```python
from build123d import *

# Parameters (mm, degrees)
SKETCH034_R     = 2.15
PAD006_DEPTH    = 14.6
SKETCH035_R     = 1.3
HOLE_DEPTH      = 8.7
HOLE_TIPS_R     = 1.3
SKETCH036_R     = 1.3
HOLE001_DEPTH   = 8.7
HOLE001_TIPS_R  = 1.3
SKETCH037_R     = 1.3
HOLE002_DEPTH   = 9.218881
HOLE002_TIPS_R  = 1.3
CHAMFER_SIZE    = 0.99
CHAMFER011_SIZE = 0.3


with BuildPart() as part:
    # Sketch034 → Pad006 (new body, symmetric)
    with BuildSketch(Plane.XZ):
        with BuildLine():
            Line((-9.454213, -1.414214), (-8.5, -2.368427))
            Line((-8.5, -2.368427), (-8.5, -5.5))
            Line((-8.5, -5.5), (-19, -5.5))
            Line((-19, -5.5), (-20, -4.5))
            Line((-20, -4.5), (-20, 11))
            Line((-20, 11), (-19, 12))
            Line((-19, 12), (-10, 12))
            Line((-10, 12), (-9, 11))
            Line((-9, 11), (9, 11))
            Line((9, 11), (10, 12))
            Line((10, 12), (19, 12))
            Line((19, 12), (20, 11))
            Line((20, 11), (20, -4.5))
            Line((20, -4.5), (19, -5.5))
            Line((19, -5.5), (8.5, -5.5))
            Line((8.5, -5.5), (8.5, -2.368427))
            Line((8.5, -2.368427), (9.454214, -1.414214))
            ThreePointArc((9.454214, -1.414214), (9.963946, 0.546289), (8.5, 1.946381))
            Line((8.5, 1.946381), (8.5, 4))
            ThreePointArc((8.5, 4), (8.207107, 4.707107), (7.5, 5))
            Line((7.5, 5), (-7.5, 5))
            ThreePointArc((-7.5, 5), (-8.207107, 4.707107), (-8.5, 4))
            Line((-8.5, 4), (-8.5, 1.946381))
            ThreePointArc((-8.5, 1.946381), (-9.963946, 0.546289), (-9.454213, -1.414214))
        make_face()
        with Locations((-16.700254, 5)):
            Circle(SKETCH034_R, mode=Mode.SUBTRACT)
        with Locations((16.700254, 5)):
            Circle(SKETCH034_R, mode=Mode.SUBTRACT)
    extrude(amount=PAD006_DEPTH, both=True)

    # Sketch035 → Hole (cut)
    with BuildSketch(Plane.XZ.offset(14.6)):
        with Locations((-14.679528, -1.5)):
            Circle(SKETCH035_R)
        with Locations((14.679528, -1.5)):
            Circle(SKETCH035_R)
        with Locations((0, 8)):
            Circle(SKETCH035_R)
    extrude(amount=-HOLE_DEPTH, mode=Mode.SUBTRACT)

    # Hole tips → Hole tip 1 section 0
    with BuildSketch(Plane.XZ.offset(5.9), mode=Mode.PRIVATE) as hole_tip_1_s0:
        with Locations((-14.679528, -1.5)):
            Circle(HOLE_TIPS_R)
    loft([hole_tip_1_s0.sketch, Vertex(-14.679528, -4.6, -1.5)], mode=Mode.SUBTRACT)

    # Hole tips → Hole tip 2 section 0
    with BuildSketch(Plane.XZ.offset(5.9), mode=Mode.PRIVATE) as hole_tip_2_s0:
        with Locations((14.679528, -1.5)):
            Circle(HOLE_TIPS_R)
    loft([hole_tip_2_s0.sketch, Vertex(14.679528, -4.6, -1.5)], mode=Mode.SUBTRACT)

    # Hole tips → Hole tip 3 section 0
    with BuildSketch(Plane.XZ.offset(5.9), mode=Mode.PRIVATE) as hole_tip_3_s0:
        with Locations((0, 8)):
            Circle(HOLE_TIPS_R)
    loft([hole_tip_3_s0.sketch, Vertex(0, -4.6, 8)], mode=Mode.SUBTRACT)

    # Sketch036 → Hole001 (cut)
    with BuildSketch(Plane(origin=(0, 14.6, 0), x_dir=(-1, 0, 0), z_dir=(0, 1, 0))):
        with Locations((14.679528, -1.5)):
            Circle(SKETCH036_R)
        with Locations((-14.679528, -1.5)):
            Circle(SKETCH036_R)
        with Locations((0, 8)):
            Circle(SKETCH036_R)
    extrude(amount=-HOLE001_DEPTH, mode=Mode.SUBTRACT)

    # Hole001 tips → Hole001 tip 1 section 0
    with BuildSketch(Plane(origin=(0, 5.9, 0), x_dir=(-1, 0, 0), z_dir=(0, 1, 0)), mode=Mode.PRIVATE) as hole001_tip_1_s0:
        with Locations((14.679528, -1.5)):
            Circle(HOLE001_TIPS_R)
    loft([hole001_tip_1_s0.sketch, Vertex(-14.679528, 4.6, -1.5)], mode=Mode.SUBTRACT)

    # Hole001 tips → Hole001 tip 2 section 0
    with BuildSketch(Plane(origin=(0, 5.9, 0), x_dir=(-1, 0, 0), z_dir=(0, 1, 0)), mode=Mode.PRIVATE) as hole001_tip_2_s0:
        with Locations((-14.679528, -1.5)):
            Circle(HOLE001_TIPS_R)
    loft([hole001_tip_2_s0.sketch, Vertex(14.679528, 4.6, -1.5)], mode=Mode.SUBTRACT)

    # Hole001 tips → Hole001 tip 3 section 0
    with BuildSketch(Plane(origin=(0, 5.9, 0), x_dir=(-1, 0, 0), z_dir=(0, 1, 0)), mode=Mode.PRIVATE) as hole001_tip_3_s0:
        with Locations((0, 8)):
            Circle(HOLE001_TIPS_R)
    loft([hole001_tip_3_s0.sketch, Vertex(0, 4.6, 8)], mode=Mode.SUBTRACT)

    # Sketch037 → Hole002 (cut)
    with BuildSketch(Plane.XY.offset(12)):
        with Locations((-12.5, 10)):
            Circle(SKETCH037_R)
        with Locations((12.5, 10)):
            Circle(SKETCH037_R)
        with Locations((12.5, -10)):
            Circle(SKETCH037_R)
        with Locations((-12.5, -10)):
            Circle(SKETCH037_R)
    extrude(amount=-HOLE002_DEPTH, mode=Mode.SUBTRACT)

    # Hole002 tips → Hole002 tip 1 section 0
    with BuildSketch(Plane.XY.offset(2.781119), mode=Mode.PRIVATE) as hole002_tip_1_s0:
        with Locations((-12.5, 10)):
            Circle(HOLE002_TIPS_R)
    loft([hole002_tip_1_s0.sketch, Vertex(-12.5, 10, 2)], mode=Mode.SUBTRACT)

    # Hole002 tips → Hole002 tip 2 section 0
    with BuildSketch(Plane.XY.offset(2.781119), mode=Mode.PRIVATE) as hole002_tip_2_s0:
        with Locations((12.5, 10)):
            Circle(HOLE002_TIPS_R)
    loft([hole002_tip_2_s0.sketch, Vertex(12.5, 10, 2)], mode=Mode.SUBTRACT)

    # Hole002 tips → Hole002 tip 3 section 0
    with BuildSketch(Plane.XY.offset(2.781119), mode=Mode.PRIVATE) as hole002_tip_3_s0:
        with Locations((12.5, -10)):
            Circle(HOLE002_TIPS_R)
    loft([hole002_tip_3_s0.sketch, Vertex(12.5, -10, 2)], mode=Mode.SUBTRACT)

    # Hole002 tips → Hole002 tip 4 section 0
    with BuildSketch(Plane.XY.offset(2.781119), mode=Mode.PRIVATE) as hole002_tip_4_s0:
        with Locations((-12.5, -10)):
            Circle(HOLE002_TIPS_R)
    loft([hole002_tip_4_s0.sketch, Vertex(-12.5, -10, 2)], mode=Mode.SUBTRACT)

    # Chamfer
    chamfer_edges = [part.edges().sort_by_distance(p)[0] for p in [
        (14.5, 14.6, 12),
        (-14.5, 14.6, 12),
        (-14.5, -14.6, 12),
        (14.5, -14.6, 12),
    ]]
    chamfer(chamfer_edges, length=CHAMFER_SIZE)

    # Chamfer011
    chamfer011_edges = [part.edges().sort_by_distance(p)[0] for p in [
        (-13.8, -10, 12),
        (-13.8, 10, 12),
        (11.2, 10, 12),
        (11.2, -10, 12),
        (13.379528, -14.6, -1.5),
        (-15.979528, -14.6, -1.5),
        (-1.3, -14.6, 8),
        (8.977107, -14.6, -1.89132),
        (9.963946, -14.6, 0.546289),
        (-8.977107, -14.6, -1.89132),
        (-9.963946, -14.6, 0.546289),
        (14.550254, -14.6, 5),
        (-18.850254, -14.6, 5),
        (-8.977107, 14.6, -1.89132),
        (-9.963946, 14.6, 0.546289),
        (8.977107, 14.6, -1.89132),
        (9.963946, 14.6, 0.546289),
        (15.979528, 14.6, -1.5),
        (1.3, 14.6, 8),
        (-13.379528, 14.6, -1.5),
        (-18.850254, 14.6, 5),
        (14.550254, 14.6, 5),
    ]]
    chamfer(chamfer011_edges, length=CHAMFER011_SIZE)


solid = part.part
```
Verification items for the finished model (mm, model axes). A direction names the side the tool comes from. Coordinates: 2 decimals unless noted, no trailing zeros. Write each loop counter-clockwise with the first axis right and the second up, starting at its lowest first coordinate (ties: lowest second). Pieces come first, ordered by that corner, then holes. Notation, with made-up numbers: (80, -33.5) - (93, -33.5) arc R33 ccw to (93, 4.5) - close; hole circle Ø1 at (-25.75, -37.75). An arc over 180 degrees is marked (long way). Write item = value, one per line.
Q1. Go/stop test with flat-tipped pins: pin 1 Ø2.5 at (x, z) = (-14.68, -1.5) entering from +Y; pin 2 Ø2 at (x, z) = (-14.68, -1.5) entering from +Y; pin 3 Ø12 at (x, y) = (-1, -7.5) entering from -Z. Record where each tip stops, or that it passes through.
Answer:
pin_1 = 5.85
pin_2 = 5.6
pin_3 = 5
Q2. Cross-section at C-C (x = 4). Enter the section's corners in (y, z), plus the area to 3 significant figures.
Answer:
outline = (-14.6, 5) - (14.6, 5) - (14.6, 11) - (-14.6, 11) - close
area = 175 mm²
Q3. Cross-section at B-B (y = 3.75). Enter the section's corners in (x, z).
Answer:
outline = (-20, -4.5) - (-19, -5.5) - (-8.5, -5.5) - (-8.5, -2.37) - (-9.45, -1.41) arc R2 cw to (-8.5, 1.95) - (-8.5, 4) arc R1 cw to (-7.5, 5) - (7.5, 5) arc R1 cw to (8.5, 4) - (8.5, 1.95) arc R2 cw to (9.45, -1.41) - (8.5, -2.37) - (8.5, -5.5) - (19, -5.5) - (20, -4.5) - (20, 11) - (19, 12) - (10, 12) - (9, 11) - (-9, 11) - (-10, 12) - (-19, 12) - (-20, 11) - close; hole circle Ø4.3 at (-16.7, 5); hole circle Ø4.3 at (16.7, 5)
Q4. Cross-section at A-A (y = -12.5). Give the number of separate pieces and of enclosed holes in the cut face, plus the area to 3 significant figures.
Answer:
separate_pieces = 1
enclosed_holes = 5
area = 447 mm²
Q5. Material ranges on L1, parallel to Y at x = 12.5, z = 9; L2, parallel to X at y = -3, z = 0; L3, parallel to Z at x = 0, y = 10, recorded low to high. Write a range as from..to.
Answer:
L1 = -14.6..-11.3, -8.7..8.7, 11.3..14.6
L2 = -20..-10.04, 10.04..20
L3 = 5..6.7, 9.3..11
Q6. Access from +Z, -Z, +X, -X, +Y, -Y to the whole of each face (thin tool, end or side, straight path). Record for faces 1 (the face through (-15, 0, 12)), 2 (the face through (12.33, 11.29, 7.3)), 3 (the face through (10.07, 14.41, 0.58)), 4 (the face through (-8.199, -0.204, 4.715)), 5 (the face through (19.5, -0.2, -5)).
Answer:
face_1 = +Z, +X, -X, +Y, -Y
face_2 = +Z
face_3 = +Y
face_4 = -Z, +Y, -Y
face_5 = -Z, +X, +Y, -Y
Q7. Mould release check, pull along Z, two halves, no side actions. Record for faces 6 (the face through (14.42, -14.1, 11.51)), 7 (the face through (20, 0, 3)), 8 (the face through (9.97, -0.2, 0.52)): released by +Z, released by -Z, zero draft, split by the parting line, or undercut.
Answer:
face_6 = released by +Z
face_7 = zero draft
face_8 = undercut
